The listing builds one solid part. Answer for the finished solid, in the listing's coordinates (mm). A direction names the side the tool comes from. Give positions to 0.01 mm unless a question says otherwise; leave off trailing zeros. Order: outer loops, then holes, each group sorted by start corner. A loop starts at its lowest first (then second) coordinate and runs counter-clockwise, first axis right, second up. Notation, with made-up numbers: (9.25, 71) - (54.25, 71) arc R29 ccw to (54.25, 102) - close; hole circle Ø2 at (42, 65). An arc over 180 degrees is marked (long way). Use a Markdown table: item, result. Add a question column.
1) Flat-ended cylindrical pins translate along their axes: pin 1 (12 mm diameter, centred on x = -2.5, z = -19.5, fed in from +Y); pin 2 (2 mm diameter, centred on x = -17.5, y = 33.5, fed in from +Z). Find the tip coordinate at first contact, or state that the pin passes through.
2) Straight lines are drawn through the part: line 1 (X direction, y = -26, z = -17); line 2 (Z direction, x = -41.5, y = 36). For each, find the intervals that lie inside material, in ascending order.
3) Find section A-A, the plane z = -20.5. Determine the outline of the cut face in (x, y).
4) Find section B-B, the plane y = 5.5. Determine the outline of the cut face in (x, z).
5) Find section C-C, the plane x = -17. Determine the outline of the cut face in (y, z).
6) For faces 4 (the face through (-1, -1, -25.405)), 5 (the face through (-119.893, -1, -25)), determine the directions among +Z, -Z, +X, -X, +Y, -Y from which every point of the face is accessible in a straight line to the end or side of a thin tool.
7) The mould has two halves that part along X. Classify faces 1 (the face through (-44.45, -1, -16)), 2 (the face through (130.107, -1, -25)), 3 (the face through (-83, 1, -5.405)): released by +X, released by -X, zero draft, split by the parting line, or undercut.
from build123d import *

# Parameters (mm, degrees)
F0_W     = 250
F0_H     = 18.0115271627
F1_DEPTH = 50
F2_W     = 75.4434949934
F2_H     = 100
F2_W_2   = 85.6565050066
F3_DEPTH = 20


with BuildPart() as f1:
    # F0 (on Front) → F1 (new body, symmetric)
    with BuildSketch(Plane.XZ):
        with Locations((5.1065050066, -34.4105418772)):
            Rectangle(F0_W, F0_H)
    extrude(amount=F1_DEPTH, both=True)

    # F2 (on face) → F3 (join)
    with BuildSketch(Plane.XY.offset(-25.4047782958)):
        with Locations((-82.1717474967, 0)):
            Rectangle(F2_W, F2_H)
        with Locations((87.2782525033, 0)):
            Rectangle(F2_W_2, F2_H)
    extrude(amount=F3_DEPTH)


solid = f1.part
The answers:
| question | item | result |
|---|---|---|
| 1 | pin 1 | y = 50 |
| 1 | pin 2 | z = -25.4 |
| 2 | line 1 | -119.89 to -44.45, 44.45 to 130.11 |
| 2 | line 2 | -43.42 to -25.4 |
| 3 | outline | (-119.89, -50) - (-44.45, -50) - (-44.45, 50) - (-119.89, 50) - close; (44.45, -50) - (130.11, -50) - (130.11, 50) - (44.45, 50) - close |
| 4 | outline | (-119.89, -43.42) - (130.11, -43.42) - (130.11, -5.4) - (44.45, -5.4) - (44.45, -25.4) - (-44.45, -25.4) - (-44.45, -5.4) - (-119.89, -5.4) - close |
| 5 | outline | (-50, -43.42) - (50, -43.42) - (50, -25.4) - (-50, -25.4) - close |
| 6 | face 4 | +Z, +Y, -Y |
| 6 | face 5 | +Z, -Z, -X, +Y, -Y |
| 7 | face 1 | undercut |
| 7 | face 2 | released by +X |
| 7 | face 3 | zero draft |
